from build123d import *

# Parameters (mm, degrees)
BOSS_EXTRUDE1_DEPTH             = 15
H_0_266_DIAMETER_HOLE1_D        = 6.7564
SKETCH5_W                       = 60
SKETCH5_H                       = 16
SKETCH5_H_2                     = 20.916111238
CUT_EXTRUDE1_DEPTH              = 74.143694192
BOSS_EXTRUDE2_REACH             = 70.374
SKETCH6_R                       = 3.3782
BOSS_EXTRUDE2_DIRECTION_2_REACH = 70.374


with BuildPart() as part:
    # Sketch1 → Boss-Extrude1 (new, symmetric)
    with BuildSketch(Plane.XY):
        with BuildLine():
            Line((-50, 15), (50, 15))
            ThreePointArc((50, 15), (65, 0), (50, -15))
            Line((50, -15), (-50, -15))
            ThreePointArc((-50, -15), (-65, 0), (-50, 15))
        make_face()
    extrude(amount=BOSS_EXTRUDE1_DEPTH, both=True)

    # H (0.266) Diameter Hole1 (through all)
    with Locations(Plane.XY.offset(15)):
        with Locations((-50, 0), (50, 0)):
            Hole(H_0_266_DIAMETER_HOLE1_D / 2)

    # Sketch5 → Cut-Extrude1 (cut, through all)
    with BuildSketch(Plane(origin=(0, 15, 0), x_dir=(1, 0, 0), z_dir=(0, 1, 0))):
        with Locations((-35, 0)):
            Rectangle(SKETCH5_W, SKETCH5_H)
        with Locations((65, 18.458055619)):
            Rectangle(SKETCH5_W, SKETCH5_H_2)
        with Locations((65, -18.458055619)):
            Rectangle(SKETCH5_W, SKETCH5_H_2)
    extrude(amount=-CUT_EXTRUDE1_DEPTH, mode=Mode.SUBTRACT)

    # Boss-Extrude2: up to this face of the body (flat: up to its plane)
    boss_extrude2_end = Plane(part.part.faces().sort_by_distance((-12.991398112, 0, 15))[0])
    # Sketch6 → Boss-Extrude2 (add, up to the picked face)
    with BuildSketch(Plane.XY, mode=Mode.PRIVATE) as boss_extrude2_sk1:
        with Locations((50, 0)):
            Circle(SKETCH6_R)
    boss_extrude2_tool1 = split(extrude(boss_extrude2_sk1.sketch, amount=BOSS_EXTRUDE2_REACH, mode=Mode.PRIVATE), bisect_by=boss_extrude2_end, keep=Keep.BOTH, mode=Mode.PRIVATE)
    add(boss_extrude2_tool1.solids().sort_by(Axis((50, 0, 0), (0, 0, 1)))[0])

    # Boss-Extrude2 direction 2: up to this face of the body (flat: up to its plane)
    boss_extrude2_direction_2_end = Plane(part.part.faces().sort_by_distance((-12.991398112, 0, -15))[0])
    # Sketch6 → Boss-Extrude2 direction 2 (add, up to the picked face)
    with BuildSketch(Plane.XY, mode=Mode.PRIVATE) as boss_extrude2_direction_2_sk1:
        with Locations((50, 0)):
            Circle(SKETCH6_R)
    boss_extrude2_direction_2_tool1 = split(extrude(boss_extrude2_direction_2_sk1.sketch, amount=-BOSS_EXTRUDE2_DIRECTION_2_REACH, mode=Mode.PRIVATE), bisect_by=boss_extrude2_direction_2_end, keep=Keep.BOTH, mode=Mode.PRIVATE)
    add(boss_extrude2_direction_2_tool1.solids().sort_by(Axis((50, 0, 0), (0, 0, -1)))[0])


solid = part.part
Work out the finished part from the listing and answer in its coordinate system (mm). A direction names the side the tool comes from. Round coordinates to 2 decimals unless told otherwise and drop trailing zeros. Write each loop counter-clockwise with the first axis right and the second up, starting at its lowest first coordinate (ties: lowest second). Pieces come first, ordered by that corner, then holes.
1) A tool of negligible diameter and unlimited length cuts with its end or side. For faces 4 (the flat face through (35, 0, -11)), 5 (the flat face through (35, 0, 12)), 6 (the cylindrical face through (46.625, 0.149, 11.451)), 7 (the flat face through (-35, 0, -8)), from which of +Z, -Z, +X, -X, +Y, -Y can it reach the whole face along a straight path? Write none if from no direction.
2) Given pin 1 Ø8 at (y, z) = (-10, 1.5) entering from +X; pin 2 Ø1.5 at (x, y) = (45, 2) entering from +Z; pin 3 Ø2 at (y, z) = (7.5, 10) entering from +X, each flat-ended and moving along its own axis, determine where each tip first touches the part or whether it passes through.
3) A cutting plane is placed at D-D (z = -3). Give the vertices of the cut face in (x, y).
4) A cutting plane is placed at B-B (y = 0). Give the vertices of the cut face in (x, z), plus the area to 3 significant figures.
5) The mould has two halves that part along X. Classify faces 1 (the cylindrical face through (46.625, 0.149, -11.451)), 2 (the flat face through (-35, 0, 8)), 3 (the flat face through (-5, 0, 0)): pulls with the +X half, pulls with the -X half, needs draft (parallel to the pull), parting line crosses it, or undercut.
6) A cutting plane is placed at A-A (z = -13). Give the vertices of the cut face in (x, y), plus the area to 3 significant figures.
7) Straight lines are drawn through the part: line 1 (Y direction, x = -50, z = 10.5); line 2 (Z direction, x = -49, y = -8); line 3 (X direction, y = -3, z = 13.75). For each, find the intervals that lie inside material, in ascending order.
8) A cutting plane is placed at C-C (x = -9). Give the vertices of the cut face in (y, z), plus the area to 3 significant figures.
Completed:
1. face 4: -Z, +Y, -Y
1. face 5: +Z, +Y, -Y
1. face 6: +Z
1. face 7: -X, +Y, -Y
2. pin 1: stops at x = 63.75
2. pin 2: stops at z = 8
2. pin 3: stops at x = 35
3. outline: (-5, -15) - (50, -15) arc R15 ccw to (50, 15) - (-5, 15) - close
4. outline: (-65, -15) - (-53.38, -15) - (-53.38, -8) - (-65, -8) - close; (-65, 8) - (-53.38, 8) - (-53.38, 15) - (-65, 15) - close; (-46.62, -15) - (35, -15) - (35, -8) - (46.62, -8) - (46.62, -15) - (53.38, -15) - (53.38, -8) - (65, -8) - (65, 8) - (53.38, 8) - (53.38, 15) - (46.62, 15) - (46.62, 8) - (35, 8) - (35, 15) - (-46.62, 15) - (-46.62, 8) - (-5, 8) - (-5, -8) - (-46.62, -8) - close
4. area: 2,520 mm2
5. face 1: undercut
5. face 2: needs draft
5. face 3: pulls with the -X half
6. outline: (-50, -15) - (35, -15) - (35, 15) - (-50, 15) arc R15 ccw to start; circle Ø6.76 at (50, 0); hole circle Ø6.76 at (-50, 0)
6. area: 2,900 mm2
7. line 1: y = -15 to -3.38, 3.38 to 15
7. line 2: z = -15 to -8, 8 to 15
7. line 3: x = -64.7 to -51.55, -48.45 to 35, 48.45 to 51.55
8. outline: (-15, -15) - (15, -15) - (15, -8) - (-15, -8) - close; (-15, 8) - (15, 8) - (15, 15) - (-15, 15) - close
8. area: 420 mm2
